```python
from build123d import *

# Parameters (mm, degrees)
SKETCH3_W            = 55.1053
SKETCH3_H            = 45.5803
BOSS_EXTRUDE2_DEPTH  = 44.45
SKETCH11_W           = 51.1175
SKETCH11_H           = 41.5925
SKETCH11_W_2         = 47.9425
SKETCH11_H_2         = 38.4175
BOSS_EXTRUDE3_DEPTH  = 3.175
SKETCH13_W           = 44.7675
SKETCH13_H           = 35.2425
CUT_EXTRUDE3_DEPTH   = 73.294764944
CUT_EXTRUDE4_DEPTH   = 5.1689
SKETCH19_W           = 1.5875
SKETCH19_H           = 45.5803
BOSS_EXTRUDE4_DEPTH  = 44.45
SKETCH21_W           = 1.5875
SKETCH21_H           = 35.2425
CUT_EXTRUDE5_DEPTH   = 39.37
FILLET1_R            = 482.6
FILLET2_R            = 482.6
SKETCH22_R           = 1.524
CUT_EXTRUDE7_DEPTH   = 3.175
BOSS_EXTRUDE5_DEPTH  = 38.1
SKETCH39_R           = 1.27
CUT_EXTRUDE14_DEPTH  = 3.81
BOSS_EXTRUDE22_DEPTH = 8.89
SKETCH48_W           = 18.288
SKETCH48_H           = 29.21
BOSS_EXTRUDE23_DEPTH = 1.5875


with BuildPart() as part:
    # Sketch3 → Boss-Extrude2 (new body)
    with BuildSketch(Plane(origin=(0, 0, 0), x_dir=(1, 0, 0), z_dir=(0, 1, 0))):
        with Locations((6.69887245, -22.79015)):
            Rectangle(SKETCH3_W, SKETCH3_H)
    extrude(amount=BOSS_EXTRUDE2_DEPTH)

    # Sketch11 → Boss-Extrude3 (add)
    with BuildSketch(Plane(origin=(0, 44.45, 0), x_dir=(1, 0, 0), z_dir=(0, 1, 0))):
        with Locations((6.69887245, -22.79015)):
            Rectangle(SKETCH11_W, SKETCH11_H)
        with Locations((6.69887245, -22.79015)):
            Rectangle(SKETCH11_W_2, SKETCH11_H_2, mode=Mode.SUBTRACT)
    extrude(amount=BOSS_EXTRUDE3_DEPTH)

    # Sketch13 → Cut-Extrude3 (cut, through all)
    with BuildSketch(Plane(origin=(0, 44.45, 0), x_dir=(1, 0, 0), z_dir=(0, 1, 0))):
        with Locations((6.69887245, -22.79015)):
            Rectangle(SKETCH13_W, SKETCH13_H)
    extrude(amount=-CUT_EXTRUDE3_DEPTH, mode=Mode.SUBTRACT)

    # Sketch14 → Cut-Extrude4 (cut)
    with BuildSketch(Plane.XY.offset(45.5803)):
        with BuildLine():
            Line((-2.82612755, 6.35), (-2.82612755, 0))
            Line((-2.82612755, 0), (3.52387245, 0))
            Line((3.52387245, 0), (3.52387245, 6.35))
            ThreePointArc((3.52387245, 6.35), (0.34887245, 9.525), (-2.82612755, 6.35))
        make_face()
        with BuildLine():
            Line((9.87387245, 6.35), (9.87387245, 0))
            Line((9.87387245, 0), (16.22387245, 0))
            Line((16.22387245, 0), (16.22387245, 6.35))
            ThreePointArc((16.22387245, 6.35), (13.04887245, 9.525), (9.87387245, 6.35))
        make_face()
        with BuildLine():
            Line((25.618069301, 0), (29.87637245, 0))
            Line((29.87637245, 0), (29.87637245, 5.08))
            ThreePointArc((29.87637245, 5.08), (27.747220876, 7.209151575), (25.618069301, 5.08))
            Line((25.618069301, 5.08), (25.618069301, 0))
        make_face()
    extrude(amount=-CUT_EXTRUDE4_DEPTH, mode=Mode.SUBTRACT)

    # Sketch19 → Boss-Extrude4 (add)
    with BuildSketch(Plane.XZ):
        with Locations((-21.64752755, 22.79015)):
            Rectangle(SKETCH19_W, SKETCH19_H)
        with Locations((35.04527245, 22.79015)):
            Rectangle(SKETCH19_W, SKETCH19_H)
    extrude(amount=-BOSS_EXTRUDE4_DEPTH)

    # Sketch21 → Cut-Extrude5 (cut)
    with BuildSketch(Plane(origin=(0, 0, 0), x_dir=(-1, 0, 0), z_dir=(0, -1, 0))):
        with Locations((16.47862755, -22.79015)):
            Rectangle(SKETCH21_W, SKETCH21_H)
        with Locations((-29.87637245, -22.79015)):
            Rectangle(SKETCH21_W, SKETCH21_H)
    extrude(amount=-CUT_EXTRUDE5_DEPTH, mode=Mode.SUBTRACT)

    # Fillet1
    # the kernel refuses this fillet: 482.6 mm, written as the material it adds along each edge
    with BuildSketch(Plane(origin=(-17.27237755, 39.37, 40.4114), x_dir=(1, 0, 0), z_dir=(0, 0, -1))) as fillet1_piece_1:
        with BuildLine():
            CenterArc((482.6, 39.111824858), FILLET1_R, 180, 4.648576264)
            Line((0, 39.111824858), (0, 0))
            Line((0, 0), (1.5875, 0))
        make_face()
    extrude(amount=35.2425)

    # Fillet2
    # the kernel refuses this fillet: 482.6 mm, written as the material it adds along each edge
    with BuildSketch(Plane(origin=(30.67012245, 39.37, 138.190962146), x_dir=(0, -1, 0), z_dir=(0, 0, -1))) as fillet2_piece_1_section:
        with BuildLine():
            CenterArc((39.111824858, 482.6), FILLET2_R, 265.351423736, 4.648576264)
            Line((0, 1.5875), (0, 0))
            Line((0, 0), (39.111824858, 0))
        make_face()
    fillet2_piece_1 = extrude(amount=230.801624292, mode=Mode.PRIVATE)
    fillet2_piece_1 = split(fillet2_piece_1, bisect_by=Plane(origin=(30.67012245, 39.37, 45.5803), z_dir=(0, 0, -1)), keep=Keep.TOP, mode=Mode.PRIVATE)
    fillet2_piece_1 = split(fillet2_piece_1, bisect_by=Plane(origin=(30.67012245, 39.37, 0), z_dir=(0, 0, 1)), keep=Keep.TOP, mode=Mode.PRIVATE)
    add(fillet2_piece_1)

    # Sketch22 → Cut-Extrude7 (cut)
    with BuildSketch(Plane.XZ):
        with Locations(Location((-19.39327755, 42.5323, 0), (0, 0, 270))):
            Circle(SKETCH22_R)
        with Locations(Location((32.79102245, 42.5323, 0), (0, 0, 270))):
            Circle(SKETCH22_R)
        with Locations(Location((-19.39327755, 3.048, 0), (0, 0, 270))):
            Circle(SKETCH22_R)
        with Locations(Location((32.79102245, 3.048, 0), (0, 0, 270))):
            Circle(SKETCH22_R)
    extrude(amount=-CUT_EXTRUDE7_DEPTH, mode=Mode.SUBTRACT)

    # Sketch23 → Boss-Extrude5 (add)
    with BuildSketch(Plane.XZ):
        with BuildLine():
            Line((24.85987245, 63.8683), (-11.46212755, 63.8683))
            add(Edge.make_bspline(
                [(-11.46212755, 63.8683), (-22.44127755, 63.8683), (-22.44127755, 58.2803)],
                knots=[4.71238898, 4.71238898, 4.71238898, 6.283185307, 6.283185307, 6.283185307], degree=2, weights=[1, 0.707106781, 1]))
            Line((-22.44127755, 58.2803), (-22.44127755, 45.5803))
            Line((-22.44127755, 45.5803), (-20.85377755, 45.5803))
            Line((-20.85377755, 45.5803), (-11.46212755, 45.5803))
            Line((-11.46212755, 45.5803), (-11.46212755, 62.2808))
            Line((-11.46212755, 62.2808), (24.85987245, 62.2808))
            Line((24.85987245, 62.2808), (24.85987245, 63.8683))
        make_face()
    extrude(amount=-BOSS_EXTRUDE5_DEPTH)

    # Sketch39 → Cut-Extrude14 (cut)
    with BuildSketch(Plane.XY.offset(63.8683)):
        with Locations((6.69887245, 35.56)):
            Circle(SKETCH39_R)
        with Locations((-6.76312755, 35.56)):
            Circle(SKETCH39_R)
        with Locations((20.16087245, 35.56)):
            Circle(SKETCH39_R)
    extrude(amount=-CUT_EXTRUDE14_DEPTH, mode=Mode.SUBTRACT)

    # Sketch43 → Boss-Extrude22 (add)
    with BuildSketch(Plane.XZ):
        with BuildLine():
            Line((31.20987245, 45.5803), (35.83902245, 45.5803))
            Line((35.83902245, 45.5803), (35.83902245, 58.2803))
            add(Edge.make_bspline(
                [(35.83902245, 58.2803), (35.83902245, 63.8683), (24.85987245, 63.8683)],
                knots=[3.141592654, 3.141592654, 3.141592654, 4.71238898, 4.71238898, 4.71238898], degree=2, weights=[1, 0.707106781, 1]))
            Line((24.85987245, 63.8683), (24.85987245, 62.2808))
            Line((24.85987245, 62.2808), (23.27237245, 62.2808))
            Line((23.27237245, 62.2808), (23.27237245, 45.5803))
            Line((23.27237245, 45.5803), (24.85987245, 45.5803))
            Line((24.85987245, 45.5803), (24.85987245, 58.2803))
            Line((24.85987245, 58.2803), (31.20987245, 58.2803))
            Line((31.20987245, 58.2803), (31.20987245, 45.5803))
        make_face()
    extrude(amount=-BOSS_EXTRUDE22_DEPTH)

    # Sketch48 → Boss-Extrude23 (add)
    with BuildSketch(Plane(origin=(24.85987245, 0, 0), x_dir=(0, 0, -1), z_dir=(1, 0, 0))):
        with Locations((-54.7243, 23.495)):
            Rectangle(SKETCH48_W, SKETCH48_H)
    extrude(amount=-BOSS_EXTRUDE23_DEPTH)


solid = part.part
```
Could you check a few things on this model? Use its own coordinates, in mm. A direction names the side the tool comes from. Give positions to 0.01 mm unless a question says otherwise; leave off trailing zeros. Loops run counter-clockwise (first coordinate to the right, second up) from the corner with the lowest first, then second, coordinate; pieces in that order, holes last. Notation, with made-up numbers: (13, 84.25) -> (66, 84.25) arc R8 ccw to (66, 93.25) -> close; hole circle Ø7 at (-16, 12.25). An arc over 180 degrees is marked (long way). Put each result on its own line as item: value.
(1) For faces 4 (the face through (32.258, 46, 23)), 5 (the face through (-2.826, 3, 43)), 6 (the face through (14, 27, 45.58)), which set-ups out of +Z, -Z, +X, -X, +Y, -Y let a thin tool reach every point of the face, with its end or its side?
Computed:
face 4: +Z, -Z, +X, +Y
face 5: -Y
face 6: +Y
(2) Imagine slicing it at C-C on z = 6.5. Write out the boundary of the cut face in (x, y) (3 decimals).
Computed:
outline: (-22.441, 0) -> (-17.272, 0) -> (-17.272, 0.258) arc R482.6 cw to (-15.685, 39.37) -> (-15.685, 44.45) -> (-17.272, 44.45) -> (-17.272, 47.625) -> (-18.86, 47.625) -> (-18.86, 44.45) -> (-22.441, 44.45) -> close; (29.083, 39.37) arc R482.6 cw to (30.67, 0.258) -> (30.67, 0) -> (35.839, 0) -> (35.839, 44.45) -> (32.258, 44.45) -> (32.258, 47.625) -> (30.67, 47.625) -> (30.67, 44.45) -> (29.083, 44.45) -> close
(3) Imagine slicing it at A-A on z = 50.5. Write out the boundary of the cut face in (x, y), plus the area to 3 significant figures.
Computed:
outline: (-22.44, 0) -> (-11.46, 0) -> (-11.46, 38.1) -> (-22.44, 38.1) -> close; (23.27, 0) -> (24.86, 0) -> (24.86, 38.1) -> (23.27, 38.1) -> close; (31.21, 0) -> (35.84, 0) -> (35.84, 8.89) -> (31.21, 8.89) -> close
area: 520 mm^2
(4) Imagine slicing it at B-B on y = 41.5. Write out the boundary of the cut face in (x, z).
Computed:
outline: (-22.44, 0) -> (35.84, 0) -> (35.84, 45.58) -> (-22.44, 45.58) -> close; hole (-15.68, 5.17) -> (29.08, 5.17) -> (29.08, 40.41) -> (-15.68, 40.41) -> close
(5) Please list where these lines run through material, in increasing order: probe 1 along Z at (x, y) = (6, 8); probe 2 along X at (y, z) = (11, 50.5); probe 3 along Z at (x, y) = (-12, 26). Write a range as [from, to].
Computed:
probe 1: [0, 5.17], [40.41, 45.58], [62.28, 63.87]
probe 2: [-22.44, -11.46], [23.27, 24.86]
probe 3: [0, 5.17], [40.41, 63.86]
(6) I'm going to push flat-ended pins straight in: pin 1 Ø3 at (x, z) = (-14, 18) entering from +Y; pin 2 Ø12 at (x, z) = (31.5, 55.5) entering from +Y; pin 3 Ø18.5 at (y, z) = (25.5, 56.5) entering from +X; pin 4 Ø2.5 at (y, z) = (46.5, 23.5) entering from -X. Where does each tip first touch, or does it pass through?
Computed:
pin 1: through
pin 2: y = 8.89
pin 3: x = 24.86
pin 4: x = -18.86
(7) Imagine slicing it at D-D on x = 2.5. Write out the boundary of the cut face in (y, z) (3 decimals), plus the area to 3 significant figures.
Computed:
outline: (0, 0) -> (44.45, 0) -> (44.45, 1.994) -> (47.625, 1.994) -> (47.625, 3.581) -> (44.45, 3.581) -> (44.45, 5.169) -> (0, 5.169) -> close; (0, 62.281) -> (38.1, 62.281) -> (38.1, 63.868) -> (0, 63.868) -> close; (8.685, 40.411) -> (44.45, 40.411) -> (44.45, 41.999) -> (47.625, 41.999) -> (47.625, 43.586) -> (44.45, 43.586) -> (44.45, 45.58) -> (8.685, 45.58) -> close
area: 485 mm^2
(8) Thinking about a two-plate mould opening in Z: for faces 1 (the face through (-22.441, 22, 30)), 2 (the face through (6, 46, 43.586)), 3 (the face through (6, 46, 41.999)), which applies, pulls with the +Z half, pulls with the -Z half, needs draft (parallel to the pull), parting line crosses it, or undercut?
Computed:
face 1: needs draft
face 2: pulls with the +Z half
face 3: undercut
